Geometry: final body of the model. Coordinates: model frame, mm. Face numbers are marked on the shaded views. Coordinates: 2 decimals unless noted, no trailing zeros. Loops run counter-clockwise (first coordinate to the right, second up) from the corner with the lowest first, then second, coordinate; pieces in that order, holes last. Notation, with made-up numbers: (-15, -37) - (31, -37) arc R27 cw to (31, -6) - close; hole circle Ø10 at (-38, 35). An arc over 180 degrees is marked (long way). Answer in a Markdown table with one row per item.
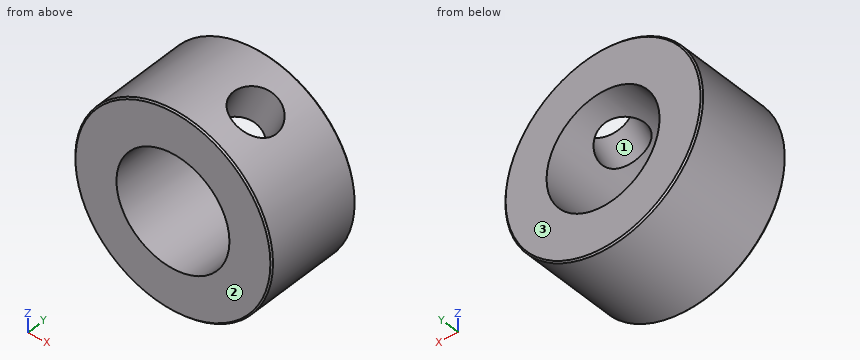
from build123d import *

# Parameters (mm, degrees)
SKETCH2_R                 = 7
SKETCH2_R_2               = 4
BOSS_EXTRUDE1_DEPTH       = 7
M4X0_7_TAPPED_HOLE1_D     = 3.3
M4X0_7_TAPPED_HOLE1_DEPTH = 4
M4X0_7_TAPPED_HOLE1_TIP   = 0.991420021
CHAMFER1_SIZE             = 0.1


with BuildPart() as part:
    # Sketch2 → Boss-Extrude1 (new body)
    with BuildSketch(Plane(origin=(0, 0, 0), x_dir=(1, 0, 0), z_dir=(0, 1, 0))):
        Circle(SKETCH2_R)
        Circle(SKETCH2_R_2, mode=Mode.SUBTRACT)
    extrude(amount=BOSS_EXTRUDE1_DEPTH)

    # M4x0.7 Tapped Hole1
    with Locations(Plane(origin=(2.919589897, 3.5, 6.362074727), x_dir=(0.908867818, 0, -0.417084271), z_dir=(0.417084271, 0, 0.908867818))):
        with Locations((0, 0)):
            Hole(M4X0_7_TAPPED_HOLE1_D / 2, depth=M4X0_7_TAPPED_HOLE1_DEPTH)
            with Locations((0, 0, -(M4X0_7_TAPPED_HOLE1_DEPTH + M4X0_7_TAPPED_HOLE1_TIP / 2))):  # 118° drill point
                Cone(0, M4X0_7_TAPPED_HOLE1_D / 2, M4X0_7_TAPPED_HOLE1_TIP, mode=Mode.SUBTRACT)

    # Chamfer1
    chamfer1_edges = [part.edges().sort_by_distance(p)[0] for p in [
        (-7, 0, 0),
        (-7, 7, 0),
    ]]
    chamfer(chamfer1_edges, length=CHAMFER1_SIZE)


solid = part.part
(1) Cut plane B-B on x = 2.5. State how many separate pieces and enclosed holes the cut face has, then the cut area to 3 significant figures.
Verdict:
| item | result |
|---|---|
| separate pieces | 3 |
| enclosed holes | 0 |
| area | 37.0 mm² |
(2) Cut plane C-C on y = 5.75. Output: boundary loops of the cut face in (x, z), then the cut area to 3 significant figures.
Verdict:
| item | result |
|---|---|
| outline | circle Ø14 at (0, 0); hole circle Ø8 at (0, 0) |
| area | 104 mm² |
(3) Cut plane A-A on z = 0. Output: boundary loops of the cut face in (x, y), then the cut area to 3 significant figures.
Verdict:
| item | result |
|---|---|
| outline | (-7, 0.1) - (-6.9, 0) - (-4, 0) - (-4, 7) - (-6.9, 7) - (-7, 6.9) - close; (4, 0) - (6.9, 0) - (7, 0.1) - (7, 6.9) - (6.9, 7) - (4, 7) - close |
| area | 42.0 mm² |
(4) Ray query, probe 1 along X at (y, z) = (3.75, 0); probe 2 along X at (y, z) = (2.75, -0.75). Return the intervals inside material, ascending.
Verdict:
| item | result |
|---|---|
| probe 1 | x = -7 to -4, 4 to 7 |
| probe 2 | x = -6.96 to -3.93, 3.93 to 6.96 |
(5) Pull-direction query (Y, two-part tool) for the marked faces 1, 2 and 3; classes: pulls with the +Y half, pulls with the -Y half, needs draft (parallel to the pull), parting line crosses it, or undercut.
Verdict:
| item | result |
|---|---|
| face 1 | undercut |
| face 2 | pulls with the -Y half |
| face 3 | pulls with the +Y half |
(6) First-contact query: pin 1 Ø6.5 at (x, z) = (0, 0) entering from -Y; pin 2 Ø1.5 at (y, z) = (4.5, -2.5) entering from +X. Flat tips, straight axial feed; report the tip coordinate or a pass-through.
Verdict:
| item | result |
|---|---|
| pin 1 | passes through |
| pin 2 | stops at x = 6.78 |
